from build123d import *

# Parameters (mm, degrees)
SKETCH1_R           = 4.25
BOSS_EXTRUDE1_DEPTH = 2
CUT_EXTRUDE1_DEPTH  = 5
CIRPATTERN1_COUNT   = 4
SKETCH3_R           = 1.5
CUT_EXTRUDE2_DEPTH  = 5
SKETCH5_R           = 1.85
CUT_EXTRUDE3_DEPTH  = 5
FILLET1_R           = 3


with BuildPart() as part:
    # Sketch1 → Boss-Extrude1 (new body)
    with BuildSketch(Plane(origin=(0, 0, 0), x_dir=(1, 0, 0), z_dir=(0, 1, 0))):
        with BuildLine():
            Line((-29, -34), (-25, -34))
            ThreePointArc((-25, -34), (-22.878679656, -33.121320344), (-22, -31))
            Line((-22, -31), (-22, -24.494897428))
            ThreePointArc((-22, -24.494897428), (-22.222539701, -23.361004009), (-22.857142857, -22.395334791))
            ThreePointArc((-22.857142857, -22.395334791), (-32, 0), (-22.857142857, 22.395334791))
            ThreePointArc((-22.857142857, 22.395334791), (-22.222539701, 23.361004009), (-22, 24.494897428))
            Line((-22, 24.494897428), (-22, 31))
            ThreePointArc((-22, 31), (-22.878679656, 33.121320344), (-25, 34))
            Line((-25, 34), (-29, 34))
            ThreePointArc((-29, 34), (-31.121320344, 34.878679656), (-32, 37))
            Line((-32, 37), (-32, 44))
            Line((-32, 44), (32, 44))
            Line((32, 44), (32, 37))
            ThreePointArc((32, 37), (31.121320344, 34.878679656), (29, 34))
            Line((29, 34), (25, 34))
            ThreePointArc((25, 34), (22.878679656, 33.121320344), (22, 31))
            Line((22, 31), (22, 24.494897428))
            ThreePointArc((22, 24.494897428), (22.222539701, 23.361004009), (22.857142857, 22.395334791))
            ThreePointArc((22.857142857, 22.395334791), (32, 0), (22.857142857, -22.395334791))
            ThreePointArc((22.857142857, -22.395334791), (22.222539701, -23.361004009), (22, -24.494897428))
            Line((22, -24.494897428), (22, -31))
            ThreePointArc((22, -31), (22.878679656, -33.121320344), (25, -34))
            Line((25, -34), (29, -34))
            ThreePointArc((29, -34), (31.121320344, -34.878679656), (32, -37))
            Line((32, -37), (32, -44))
            Line((32, -44), (-32, -44))
            Line((-32, -44), (-32, -37))
            ThreePointArc((-32, -37), (-31.121320344, -34.878679656), (-29, -34))
        make_face()
        with Locations(Location((0, 0, 0), (0, 0, 270))):
            Circle(SKETCH1_R, mode=Mode.SUBTRACT)
    extrude(amount=BOSS_EXTRUDE1_DEPTH)

    # Sketch2 → Cut-Extrude1 (cut)
    with BuildSketch(Plane(origin=(0, 2, 0), x_dir=(1, 0, 0), z_dir=(0, 1, 0))):
        with BuildLine():
            ThreePointArc((-11.674129624, 22.106892534), (-9.194159134, 22.25327912), (-7.454156207, 20.48012586))
            Line((-7.454156207, 20.48012586), (-6.070255366, 16.677889548))
            ThreePointArc((-6.070255366, 16.677889548), (-6.073907786, 14.615788781), (-7.40777769, 13.043190932))
            ThreePointArc((-7.40777769, 13.043190932), (-10.606601718, 10.606601718), (-13.043190932, 7.40777769))
            ThreePointArc((-13.043190932, 7.40777769), (-14.615788781, 6.073907786), (-16.677889548, 6.070255366))
            Line((-16.677889548, 6.070255366), (-20.48012586, 7.454156207))
            ThreePointArc((-20.48012586, 7.454156207), (-22.25327912, 9.194159134), (-22.106892534, 11.674129624))
            ThreePointArc((-22.106892534, 11.674129624), (-17.67766953, 17.67766953), (-11.674129624, 22.106892534))
        make_face()
    cut_extrude1 = extrude(amount=-CUT_EXTRUDE1_DEPTH, mode=Mode.SUBTRACT)

    # CirPattern1: Cut-Extrude1 ×4 about axis
    cirpattern1_axis = Axis((0, 0, 0), (0, 1, 0))
    for i in range(1, CIRPATTERN1_COUNT):
        add(cut_extrude1.rotate(cirpattern1_axis, i * 360 / CIRPATTERN1_COUNT), mode=Mode.SUBTRACT)

    # Sketch3 → Cut-Extrude2 (cut)
    with BuildSketch(Plane(origin=(0, 2, 0), x_dir=(1, 0, 0), z_dir=(0, 1, 0))):
        with Locations(Location((-8.5, 0, 0), (0, 0, 270))):
            Circle(SKETCH3_R)
        with Locations(Location((8.5, 0, 0), (0, 0, 270))):
            Circle(SKETCH3_R)
    extrude(amount=-CUT_EXTRUDE2_DEPTH, mode=Mode.SUBTRACT)

    # Sketch5 → Cut-Extrude3 (cut)
    with BuildSketch(Plane(origin=(0, 2, 0), x_dir=(1, 0, 0), z_dir=(0, 1, 0))):
        with Locations(Location((25, 38.82, 0), (0, 0, 270))):
            Circle(SKETCH5_R)
        with Locations(Location((-25, 38.82, 0), (0, 0, 270))):
            Circle(SKETCH5_R)
        with Locations(Location((-25, -38.82, 0), (0, 0, 270))):
            Circle(SKETCH5_R)
        with Locations(Location((25, -38.82, 0), (0, 0, 270))):
            Circle(SKETCH5_R)
    extrude(amount=-CUT_EXTRUDE3_DEPTH, mode=Mode.SUBTRACT)

    # Fillet1
    fillet1_edges = [part.edges().sort_by_distance(p)[0] for p in [
        (-32, 1, -44),
        (32, 1, -44),
        (32, 1, 44),
        (-32, 1, 44),
    ]]
    fillet(fillet1_edges, radius=FILLET1_R)


solid = part.part
Verification items for the finished model (mm, model axes). A direction names the side the tool comes from. Coordinates: 2 decimals unless noted, no trailing zeros. Loops run counter-clockwise (first coordinate to the right, second up) from the corner with the lowest first, then second, coordinate; pieces in that order, holes last. Notation, with made-up numbers: (1, -22) -> (52, -22) arc R26 ccw to (52, 13) -> close; hole circle Ø10 at (71.5, 45.5). An arc over 180 degrees is marked (long way). Answer as a JSON object with one key per item and string values. Group by question number.
Item 1: Scan lines: probe 1 along X at (y, z) = (1.4, -38.82); probe 2 along Z at (x, y) = (-23.5, 0.5); probe 3 along X at (y, z) = (0.25, 11). Record each from-to range of solid material in increasing order.
Item 2: Sectioned sample at A-A on x = 19. Record the boundary of the cut face in (y, z), plus the area to 3 significant figures.
Item 3: Mould release check, pull along X, two halves, no side actions. Record for faces 4 (the flat face through (0, 1, -44)), 5 (the cylindrical face through (-23.166, 1.014, -39.061)), 6 (the flat face through (-22, 1, -28)): +X half, -X half, draft (parallel to the pull), parting line (faces both ways), or undercut.
Item 4: Sectioned sample at D-D on y = 1.5. State how many separate pieces and enclosed holes the cut face has, plus the area to 3 significant figures.
Item 5: Sectioned sample at B-B on z = 18.5. Record the boundary of the cut face in (x, y).
Item 6: Sectioned sample at C-C on x = 8.5. Record the boundary of the cut face in (y, z).
Item 7: Tool access check on faces 1 (the cylindrical face through (-22.86, 0.99, -33.1)), 2 (the cylindrical face through (22.9, 0.99, -33.14)), 3 (the cylindrical face through (9.228, 1.014, 22.266)). Record the directions out of +Z, -Z, +X, -X, +Y, -Y that give a thin tool (end or side, any length) a straight path to the whole face; none if there is none.
Item 8: Depth check by flat-ended pin: pin 1 (2.5 mm diameter, centred on x = 8.5, z = 0, fed in from +Y); pin 2 (1 mm diameter, centred on y = 1, z = -28.5, fed in from -X); pin 3 (1 mm diameter, centred on y = 1.5, z = -27.5, fed in from +X). Enter the tip coordinate at first touch or a pass-through.
Evaluation:
{
 "1": {"probe 1": "x = -32 to -26.85, -23.15 to 23.15, 26.85 to 32", "probe 2": "z = -44 to -39.9, -37.74 to -33.6, -21.72 to 21.72, 33.6 to 37.74, 39.9 to 44", "probe 3": "x = -30.05 to -22.36, -10.2 to 10.2, 22.36 to 30.05"},
 "2": {"outline": "(0, -44) -> (2, -44) -> (2, -16.25) -> (0, -16.25) -> close; (0, -6.92) -> (2, -6.92) -> (2, 6.92) -> (0, 6.92) -> close; (0, 16.25) -> (2, 16.25) -> (2, 44) -> (0, 44) -> close", "area": "139 mm²"},
 "3": {"face 4": "draft", "face 5": "undercut", "face 6": "-X half"},
 "4": {"separate pieces": "1", "enclosed holes": "11", "area": "4,130 mm²"},
 "5": {"outline": "(-26.11, 0) -> (-16.82, 0) -> (-16.82, 2) -> (-26.11, 2) -> close; (-6.73, 0) -> (6.73, 0) -> (6.73, 2) -> (-6.73, 2) -> close; (16.82, 0) -> (26.11, 0) -> (26.11, 2) -> (16.82, 2) -> close"},
 "6": {"outline": "(0, -44) -> (2, -44) -> (2, -21.87) -> (0, -21.87) -> close; (0, -12.36) -> (2, -12.36) -> (2, -1.5) -> (0, -1.5) -> close; (0, 1.5) -> (2, 1.5) -> (2, 12.36) -> (0, 12.36) -> close; (0, 21.87) -> (2, 21.87) -> (2, 44) -> (0, 44) -> close"},
 "7": {"face 1": "-X, +Y, -Y", "face 2": "+X, +Y, -Y", "face 3": "+Y, -Y"},
 "8": {"pin 1": "passes through", "pin 2": "stops at x = -22", "pin 3": "stops at x = 22"}
}
